For this review, use the dimensioned drawing (mm, ordinates from the lowest corner) and the shaded views. Coordinates: 2 decimals unless noted, no trailing zeros. Loops run counter-clockwise (first coordinate to the right, second up) from the corner with the lowest first, then second, coordinate; pieces in that order, holes last. Notation, with made-up numbers: M 42,75 L 77,75 A22 cw 77,99 Z; hole C -31.75,78.5 d1. An arc over 180 degrees is marked long. One line per item, written item: value.
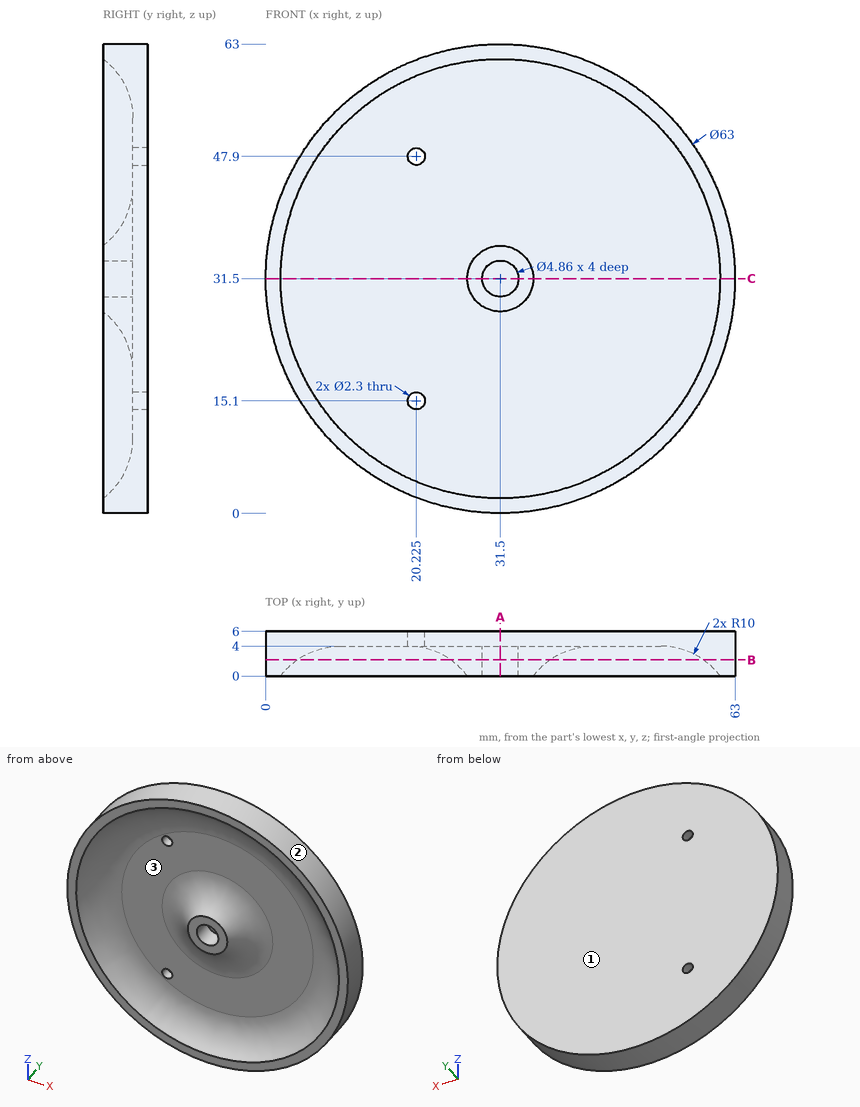
(1) Insertion check: pin 1 Ø2 at (y, z) = (2, 39.5) entering from +X; pin 2 Ø1.4 at (x, z) = (20.225, 15.1) entering from -Y. Each pin has a flat end and moves straight along its axis. Give the tip position at first contact, or say it passes through.
Checks:
pin 1: x = 62.21
pin 2: through
(2) Add section B-B on y = 2.15. State the section outline as (x, z) points, then the cut area to 3 significant figures.
Checks:
outline: C 31.5,31.5 d63; C 31.5,31.5 d13.27; hole C 31.5,31.5 d54.59; hole C 31.5,31.5 d4.86
area: 897 mm^2
(3) Add section A-A on x = 31.5. State the section outline as (y, z) points.
Checks:
outline: M 0,0 L 6,0 L 6,63 L 0,63 L 0,61 A10 cw 4,53 L 4,43.93 A10 cw 0,35.93 L 0,33.93 L 4,33.93 L 4,29.07 L 0,29.07 L 0,27.07 A10 cw 4,19.07 L 4,10 A10 cw 0,2 Z
(4) To check wall thickness, follow L1, parallel to X at y = 2.5, z = 31.5; L2, parallel to X at y = 2.2, z = 31.5; L3, parallel to Y at x = 42, z = 44.5. State the ranges of each line that lie inside material, in increasing order. Write a range as [from, to].
Checks:
L1: [0, 4.73], [24.34, 29.07], [33.93, 38.66], [58.27, 63]
L2: [0, 4.28], [24.79, 29.07], [33.93, 38.21], [58.72, 63]
L3: [4, 6]
(5) Draft analysis for pull direction Z (two halves, no side actions). For the marked faces 1, 2 and 3, state which applies: pulls with the +Z half, pulls with the -Z half, needs draft (parallel to the pull), parting line crosses it, or undercut.
Checks:
face 1: needs draft
face 2: parting line crosses it
face 3: undercut
(6) Add section C-C on z = 31.5. State the section outline as (x, y) points, then the cut area to 3 significant figures.
Checks:
outline: M 0,0 L 2,0 A10 cw 10,4 L 19.07,4 A10 cw 27.07,0 L 29.07,0 L 29.07,4 L 33.93,4 L 33.93,0 L 35.93,0 A10 cw 43.93,4 L 53,4 A10 cw 61,0 L 63,0 L 63,6 L 0,6 Z
area: 197 mm^2
